Input: part model. Units: mm. Frame: model coordinates. Coordinates: 2 decimals unless noted, no trailing zeros. Order: outer loops, then holes, each group sorted by start corner. A loop starts at its lowest first (then second) coordinate and runs counter-clockwise, first axis right, second up. Notation, with made-up numbers: (-16, -16.75) - (17, -16.75) arc R34 ccw to (17, 18.25) - close; hole circle Ø8 at (41.25, 87). An arc over 180 degrees is marked (long way). One line per question, with ' | ' between items.
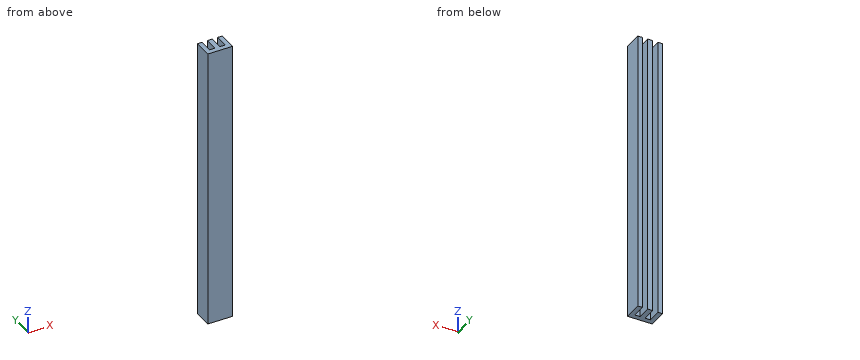
from build123d import *

# Parameters (mm, degrees)
ESBO_O1_W                = 1.8
ESBO_O1_H                = 5.5
RESSALTO_EXTRUS_O1_DEPTH = 115


with BuildPart() as part:
    # Esboço1 → Ressalto-extrusão1 (new body)
    with BuildSketch(Plane.XY):
        with Locations((-8.1, 1.25)):
            Rectangle(ESBO_O1_W, ESBO_O1_H)
        Polygon((-5, -1.198132677), (-5, -1.5), (-4, -1.5), (-4, 4), (-5, 4), align=None)
        Polygon((-4, 4), (-4, -1.5), (-3, -1.5), (-3, -1.198132677), (-3, 4), align=None)
        Polygon((-4, -1.5), (-5, -1.5), (-5.301867323, -1.5), (-6.898310084, -1.5), (-7.2, -1.5), (-9, -1.5), (-9, -3.5), (1, -3.5), (1, -1.5), (-0.8, -1.5), (-1.101689916, -1.5), (-2.698132677, -1.5), (-3, -1.5), align=None)
        with Locations((0.1, 1.25)):
            Rectangle(ESBO_O1_W, ESBO_O1_H)
    extrude(amount=RESSALTO_EXTRUS_O1_DEPTH)


solid = part.part
Item 1: Contact query for flat-ended pins moving along their axis: P1, Ø1.8, axis at x = -6, z = 45.5, coming from the +Y side; P2, Ø2, axis at x = -5, y = -1, coming from the -Z side. Output: stop coordinate, or through.
Data:
P1: y = -1.5 | P2: z = 0
Item 2: Section C-C on x = -2. Return the cut outline in (y, z).
Data:
outline: (-3.5, 0) - (-1.5, 0) - (-1.5, 115) - (-3.5, 115) - close
Item 3: Section A-A on y = 2.75. Return the cut outline in (x, z), and give its area (3 significant figures).
Data:
outline: (-9, 0) - (-7.2, 0) - (-7.2, 115) - (-9, 115) - close; (-5, 0) - (-3, 0) - (-3, 115) - (-5, 115) - close; (-0.8, 0) - (1, 0) - (1, 115) - (-0.8, 115) - close | area: 644 mm^2
Item 4: Section B-B on z = 26.5. Return the cut outline in (x, y), and give its area (3 significant figures).
Data:
outline: (-9, -3.5) - (1, -3.5) - (1, 4) - (-0.8, 4) - (-0.8, -1.5) - (-3, -1.5) - (-3, 4) - (-5, 4) - (-5, -1.5) - (-7.2, -1.5) - (-7.2, 4) - (-9, 4) - close | area: 50.8 mm^2
Item 5: Ray query, line 1 (X direction, y = 1, z = 90); line 2 (Y direction, x = -2.5, z = 45). Return the intervals inside material, ascending.
Data:
line 1: -9 to -7.2, -5 to -3, -0.8 to 1 | line 2: -3.5 to -1.5
